Design review of the part built by this model. Coordinates are the model's own, in mm. Face numbers are marked on the shaded views. A direction names the side the tool comes from. Coordinates: 2 decimals unless noted, no trailing zeros. Write each loop counter-clockwise with the first axis right and the second up, starting at its lowest first coordinate (ties: lowest second). Pieces come first, ordered by that corner, then holes. Notation, with made-up numbers: (16, 46.25) - (56, 46.25) arc R16 cw to (56, 62.25) - close; hole circle Ø1 at (0, 10). An arc over 180 degrees is marked (long way). Use a Markdown table: item, result.
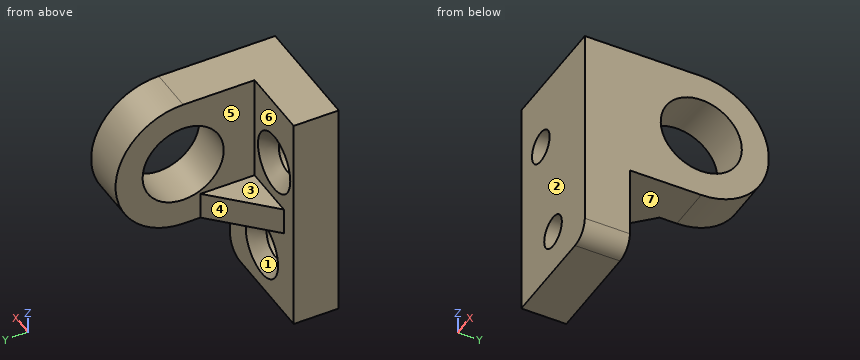
from build123d import *

# Parameters (mm, degrees)
SKETCH_1_R                = 4.5
EXTRUDE_1_DEPTH           = 5
SKETCH_2_W                = 13
SKETCH_2_H                = 25
EXTRUDE_2_DEPTH           = 5
RIB_1_REACH               = 23.352
SKETCH_3_WALL_W           = 53.190153214
SKETCH_3_WALL_H           = 3
HOLE_WIZARD_1_D           = 3.6
HOLE_WIZARD_1_CSINK_D     = 6.6
HOLE_WIZARD_1_CSINK_ANGLE = 90
FILLET_1_R                = 2


with BuildPart() as part:
    # 草图1 → 凸台-拉伸1 (new body)
    with BuildSketch(Plane(origin=(0, 0, 0), x_dir=(0, 0, -1), z_dir=(1, 0, 0))):
        with BuildLine():
            Line((7.5, 0), (7.5, -12.920004632))
            Line((7.5, -12.920004632), (-7.5, -12.920004632))
            Line((-7.5, -12.920004632), (-7.5, 0))
            ThreePointArc((-7.5, 0), (0, 7.5), (7.5, 0))
        make_face()
        Circle(SKETCH_1_R, mode=Mode.SUBTRACT)
    extrude(amount=EXTRUDE_1_DEPTH)

    # 草图2 → 凸台-拉伸2 (add)
    with BuildSketch(Plane.XZ.offset(12.920004632)):
        with Locations((-1.5, -5)):
            Rectangle(SKETCH_2_W, SKETCH_2_H)
    extrude(amount=-EXTRUDE_2_DEPTH)

    # 草图3 wall → 筋1 (add, up to next)
    with BuildSketch(Plane(origin=(-3, -4.920004632, -7.5), x_dir=(-0.707106781187, -0.707106781187, 0), z_dir=(-0.707106781187, 0.707106781187, 0)), mode=Mode.PRIVATE) as rib_1_sk1:
        with Locations((0, 1.5)):
            Rectangle(SKETCH_3_WALL_W, SKETCH_3_WALL_H)
    rib_1_tool1 = extrude(rib_1_sk1.sketch, amount=-RIB_1_REACH, mode=Mode.PRIVATE) - part.part
    add(rib_1_tool1.solids().sort_by_distance((-3, -4.920004632, -7.5))[0])

    # 打孔尺寸(%根据十字)槽半沉头木螺钉的类型1 (through all)
    with Locations(Plane(origin=(0, -7.920004632, 0), x_dir=(1, 0, 0), z_dir=(0, 1, 0))):
        with Locations((-1.5, 12.5), (-4, 0)):
            CounterSinkHole(HOLE_WIZARD_1_D / 2, HOLE_WIZARD_1_CSINK_D / 2, counter_sink_angle=HOLE_WIZARD_1_CSINK_ANGLE)

    # 圆角1
    fillet_1_edges = [part.edges().sort_by_distance(p)[0] for p in [
        (5, -10.420004632, -17.5),
    ]]
    fillet(fillet_1_edges, radius=FILLET_1_R)


solid = part.part
(1) Take a section at C-C on y = -3.25. Write out the cut boundary in (x, z).
Determined:
| item | result |
|---|---|
| outline | (-1.33, -7.5) - (5, -7.5) - (5, -3.11) - (0, -3.11) - (0, -4.5) - (-1.33, -4.5) - close; (0, 3.11) - (5, 3.11) - (5, 7.5) - (0, 7.5) - close |
(2) Draft analysis for pull direction Z (two halves, no side actions). For the marked faces 1, 2 and 3, state which applies: +Z half, -Z half, draft (parallel to the pull), parting line (faces both ways), or undercut.
Determined:
| item | result |
|---|---|
| face 1 | undercut |
| face 2 | draft |
| face 3 | +Z half |
(3) For pin 1 (7 mm diameter, centred on y = 0, z = 0, fed in from +X); pin 2 (5 mm diameter, centred on x = -0.5, y = -3.5, fed in from -Z); pin 3 (3 mm diameter, centred on x = -3.5, y = -4.5, fed in from +Z), all flat-tipped, find the tip position at first contact; note any pin that passes through.
Determined:
| item | result |
|---|---|
| pin 1 | through |
| pin 2 | z = -7.5 |
| pin 3 | z = -4.5 |
(4) Take a section at A-A on z = 0. Write out the cut boundary in (x, y), and give its area (4 significant figures).
Determined:
| item | result |
|---|---|
| outline | (-8, -12.92) - (-5.8, -12.92) - (-5.8, -9.42) - (-7.3, -7.92) - (-8, -7.92) - close; (-2.2, -12.92) - (5, -12.92) - (5, -4.5) - (0, -4.5) - (0, -7.92) - (-0.7, -7.92) - (-2.2, -9.42) - close; (0, 4.5) - (5, 4.5) - (5, 7.5) - (0, 7.5) - close |
| area | 76.85 mm2 |
(5) Machinability: for the marked faces 4, 5, 6 and 7, which of the approach directions +Z, -Z, +X, -X, +Y, -Y give a long, thin tool a straight path to every point of the face, cutting with its end or side? Answer none if there is none.
Determined:
| item | result |
|---|---|
| face 4 | +Z, -Z, -X, +Y |
| face 5 | +Z, -X, +Y |
| face 6 | -X, +Y |
| face 7 | -Z, +X, -X, +Y |
(6) Take a section at B-B on y = -10. Write out the cut boundary in (x, z), and give its area (3 significant figures).
Determined:
| item | result |
|---|---|
| outline | (-8, -17.5) - (3, -17.5) arc R2 ccw to (5, -15.5) - (5, 7.5) - (-8, 7.5) - close; hole circle Ø3.6 at (-4, 0); hole circle Ø3.6 at (-1.5, -12.5) |
| area | 304 mm2 |
(7) For L1, parallel to X at y = -10.4, z = -12.5; L2, parallel to Y at x = -7, z = -11.5; L3, parallel to Z at x = 4.25, y = -7.75, list the stretches that pass through material, from the lowest coordinate up. Write a range as from..to.
Determined:
| item | result |
|---|---|
| L1 | -8..-3.3, 0.3..5 |
| L2 | -12.92..-7.92 |
| L3 | -7.5..7.5 |
(8) Take a section at D-D on z = -7. Write out the cut boundary in (x, y), and give its area (3 significant figures).
Determined:
| item | result |
|---|---|
| outline | (-8, -12.92) - (5, -12.92) - (5, 2.69) - (0, 2.69) - (0, -1.92) - (-6, -7.92) - (-8, -7.92) - close |
| area | 136 mm2 |
